For this review, take the finished solid that the model builds, in its own axes (mm). A direction names the side the tool comes from. Give positions to 0.01 mm unless a question says otherwise; leave off trailing zeros. Write each loop counter-clockwise with the first axis right and the second up, starting at its lowest first coordinate (ties: lowest second). Pieces come first, ordered by that corner, then holes. Notation, with made-up numbers: M 9,73 L 15,73 A16 cw 15,86 Z; hole C 61.25,41.25 d10. An arc over 180 degrees is marked long. Write item = value, one per line.
```python
from build123d import *

# Parameters (mm, degrees)
F1_DEPTH = 15
F2_DEPTH = 12
F3_DEPTH = 3


with BuildPart() as f1:
    # F0 (on Front) → F1 (new body)
    with BuildSketch(Plane.XZ):
        with BuildLine():
            ThreePointArc((27.111572217, -12.8918176383), (29.93394524, -0.3222598375), (27.2243880974, 12.2720989346))
            ThreePointArc((27.2243880974, 12.2720989346), (-30.0654517858, -0.0532681334), (27.111572217, -12.8918176383))
        make_face()
        Polygon((-11.5470053838, -20), (-23.0940107676, 0), (-11.5470053838, 20), (11.5470053838, 20), (23.0940107676, 0), (11.5470053838, -20), align=None, mode=Mode.SUBTRACT)
    extrude(amount=F1_DEPTH)



with BuildPart() as f1b:
    # F0 (on Front) → F1, piece 2 (new body)
    with BuildSketch(Plane.XZ):
        with BuildLine():
            ThreePointArc((112.9235786366, -12.0569396696), (149.0649853319, -0.1668697578), (112.8282363773, 11.4293824652))
            ThreePointArc((112.8282363773, 11.4293824652), (109.0653149154, -0.3292476273), (112.9235786366, -12.0569396696))
        make_face()
        Polygon((114.7340843825, 4.5029248509), (128.9999321269, 14.8676699353), (143.2657798714, 4.5029248509), (137.8167109113, -12.2675849804), (120.1831533425, -12.2675849804), align=None, mode=Mode.SUBTRACT)
    extrude(amount=F1_DEPTH)


with BuildPart() as f1_1:
    add(f1.part)

    add(f1b.part)  # F2 merges F1b
    # F0 (on Front) → F2 (join)
    with BuildSketch(Plane.XZ):
        with BuildLine():
            Line((108.7690079407, 9.3487427546), (31.7727449925, 9.3487427546))
            ThreePointArc((31.7727449925, 9.3487427546), (29.0693414988, 10.1426032479), (27.2243880974, 12.2720989346))
            ThreePointArc((27.2243880974, 12.2720989346), (29.93394524, -0.3222598375), (27.111572217, -12.8918176383))
            ThreePointArc((27.111572217, -12.8918176383), (28.9566070835, -10.7909427918), (31.6411264653, -10.0091599138))
            Line((31.6411264653, -10.0091599138), (108.8881857649, -10.0091599138))
            ThreePointArc((108.8881857649, -10.0091599138), (111.1508057925, -10.5503988067), (112.9235786366, -12.0569396696))
            ThreePointArc((112.9235786366, -12.0569396696), (109.0653149154, -0.3292476273), (112.8282363773, 11.4293824652))
            ThreePointArc((112.8282363773, 11.4293824652), (111.0497094285, 9.8992033713), (108.7690079407, 9.3487427546))
        make_face()
        with BuildLine():
            ThreePointArc((34.9465236354, -0.3302085796), (36.4109897295, 3.2053253263), (39.9465236354, 4.6697914204))
            Line((39.9465236354, 4.6697914204), (99.9465236354, 4.6697914204))
            ThreePointArc((99.9465236354, 4.6697914204), (103.4820575413, 3.2053253263), (104.9465236354, -0.3302085796))
            ThreePointArc((104.9465236354, -0.3302085796), (103.4820575413, -3.8657424855), (99.9465236354, -5.3302085796))
            Line((99.9465236354, -5.3302085796), (39.9465236354, -5.3302085796))
            ThreePointArc((39.9465236354, -5.3302085796), (36.4109897295, -3.8657424855), (34.9465236354, -0.3302085796))
        make_face(mode=Mode.SUBTRACT)
    extrude(amount=F2_DEPTH)

    # F0 (on Front) → F3 (cut)
    with BuildSketch(Plane.XZ):
        with BuildLine():
            Line((108.7690079407, 9.3487427546), (31.7727449925, 9.3487427546))
            ThreePointArc((31.7727449925, 9.3487427546), (29.0693414988, 10.1426032479), (27.2243880974, 12.2720989346))
            ThreePointArc((27.2243880974, 12.2720989346), (29.93394524, -0.3222598375), (27.111572217, -12.8918176383))
            ThreePointArc((27.111572217, -12.8918176383), (28.9566070835, -10.7909427918), (31.6411264653, -10.0091599138))
            Line((31.6411264653, -10.0091599138), (108.8881857649, -10.0091599138))
            ThreePointArc((108.8881857649, -10.0091599138), (111.1508057925, -10.5503988067), (112.9235786366, -12.0569396696))
            ThreePointArc((112.9235786366, -12.0569396696), (109.0653149154, -0.3292476273), (112.8282363773, 11.4293824652))
            ThreePointArc((112.8282363773, 11.4293824652), (111.0497094285, 9.8992033713), (108.7690079407, 9.3487427546))
        make_face()
        with BuildLine():
            ThreePointArc((34.9465236354, -0.3302085796), (36.4109897295, 3.2053253263), (39.9465236354, 4.6697914204))
            Line((39.9465236354, 4.6697914204), (99.9465236354, 4.6697914204))
            ThreePointArc((99.9465236354, 4.6697914204), (103.4820575413, 3.2053253263), (104.9465236354, -0.3302085796))
            ThreePointArc((104.9465236354, -0.3302085796), (103.4820575413, -3.8657424855), (99.9465236354, -5.3302085796))
            Line((99.9465236354, -5.3302085796), (39.9465236354, -5.3302085796))
            ThreePointArc((39.9465236354, -5.3302085796), (36.4109897295, -3.8657424855), (34.9465236354, -0.3302085796))
        make_face(mode=Mode.SUBTRACT)
    extrude(amount=F3_DEPTH, mode=Mode.SUBTRACT)


solid = f1_1.part
```
1. The part is to be moulded in two halves that separate along Z. For faces 1 (the face through (69, -12, 5)), 2 (the face through (0, -7, -20)), 3 (the face through (28.923, -7.437, -10.812)), say which applies: +Z half, -Z half, draft (parallel to the pull), parting line (faces both ways), or undercut.
Responses:
face_1 = draft
face_2 = undercut
face_3 = -Z half
2. For line 1 along Z through (x, y) = (88.5, -11); line 2 along X through (y, z) = (-12.5, -5); line 3 along X through (y, z) = (-14.5, 7.5), list the stretches that pass through material, from the lowest coordinate up. Write a range as from..to.
Responses:
line_1 = -10.01..-5.33, 4.67..9.35
line_2 = -29.68..-20.21, 20.21..29.55, 109.64..117.82, 140.18..148.49
line_3 = -29.06..-18.76, 18.76..28.93, 110.63..118.86, 139.14..147.5
3. We need section D-D, the plane x = 9. Write out the cut boundary in (y, z), then the cut area to 3 significant figures.
Responses:
outline = M -15,-28.79 L 0,-28.79 L 0,-20 L -15,-20 Z; M -15,20 L 0,20 L 0,28.41 L -15,28.41 Z
area = 258 mm2
4. Machinability: for faces 4 (the face through (29.103, -7.437, 10.121)), 5 (the face through (70, -7, -10.009)), 6 (the face through (129, -7, -12.268)), 7 (the face through (20, 0, 7)), which of the approach directions +Z, -Z, +X, -X, +Y, -Y give a long, thin tool a straight path to every point of the face, cutting with its end or side? Answer none if there is none.
Responses:
face_4 = +Z, +Y, -Y
face_5 = -Z, +Y, -Y
face_6 = +Y, -Y
face_7 = +Z, -Z, +X, -X, +Y
5. We need section C-C, the plane z = -3. Write out the cut boundary in (x, y), then the cut area to 3 significant figures.
Responses:
outline = M -29.93,-15 L -21.36,-15 L -21.36,0 L -29.93,0 Z; M 21.36,-15 L 29.8,-15 L 29.8,-12 L 35.72,-12 L 35.72,-3 L 29.8,-3 L 29.8,0 L 21.36,0 Z; M 104.17,-12 L 109.26,-12 L 109.26,-15 L 117.17,-15 L 117.17,0 L 109.26,0 L 109.26,-3 L 104.17,-3 Z; M 140.83,-15 L 148.87,-15 L 148.87,0 L 140.83,0 Z
area = 594 mm2
6. We need section B-B, the plane y = -5. Write out the cut boundary in (x, z).
Responses:
outline = M 27.11,-12.89 A5 cw 31.64,-10.01 L 108.89,-10.01 A5 cw 112.92,-12.06 A20 ccw long 112.83,11.43 A5 cw 108.77,9.35 L 31.77,9.35 A5 cw 27.22,12.27 A30 ccw long Z; hole M -23.09,0 L -11.55,-20 L 11.55,-20 L 23.09,0 L 11.55,20 L -11.55,20 Z; hole M 39.95,-5.33 L 99.95,-5.33 A5 ccw 99.95,4.67 L 39.95,4.67 A5 ccw Z; hole M 114.73,4.5 L 120.18,-12.27 L 137.82,-12.27 L 143.27,4.5 L 129,14.87 Z
7. We need section A-A, the plane x = 79.5. Write out the cut boundary in (y, z), then the cut area to 3 significant figures.
Responses:
outline = M -12,-10.01 L -3,-10.01 L -3,-5.33 L -12,-5.33 Z; M -12,4.67 L -3,4.67 L -3,9.35 L -12,9.35 Z
area = 84.2 mm2
8. Insertion check: P1, Ø4, axis at x = 126, y = -2, coming from the -Z side; P2, Ø20, axis at x = 87, z = -4.5, coming from the +Y side; P3, Ø3, axis at x = 102, z = 0.5, coming from the -Y side; P4, Ø4, axis at x = 19, y = -4, coming from the -Z side. Each pin has a flat end and moves straight along its axis. Give the tip position at first contact, or say it passes through.
Responses:
P1 = -20.22
P2 = -3
P3 = through
P4 = -24.86
